Work out the finished part from the listing and answer in its coordinate system (mm). Face numbers are marked on the shaded views. A direction names the side the tool comes from. Coordinates: 2 decimals unless noted, no trailing zeros. Order: outer loops, then holes, each group sorted by start corner. A loop starts at its lowest first (then second) coordinate and runs counter-clockwise, first axis right, second up. Notation, with made-up numbers: M 75.5,44 L 105.5,44 A19 ccw 105.5,70 Z; hole C -24.75,65.25 d8. An arc over 180 degrees is marked long. Use a Markdown table: item, result.
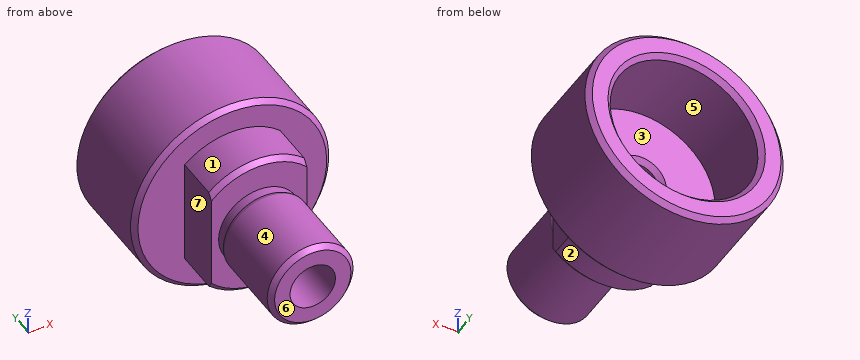
from build123d import *

# Parameters (mm, degrees)
CHAFL_N1_SIZE         = 1
REDONDEO1_R           = 1
CHAFL_N2_SIZE         = 1
CROQUIS3_W            = 14.730869345
CROQUIS3_H            = 22.360679774
CORTAR_EXTRUIR1_DEPTH = 30


with BuildPart() as part:
    # Croquis1 → Revolución1 (revolve)
    with BuildSketch(Plane.XY, mode=Mode.PRIVATE) as revoluci_n1_sk:
        Polygon((15.5, 52), (20.790206312, 52), (20.790206312, 30), (15, 30), (15, 20), (8.5, 20), (8.5, 17.951688966), (9, 17.951688966), (9, 0), (4.7625, 0), (4.7625, 30), (4.2625, 30), (4.2625, 34), (5.2625, 35), (15.5, 35), align=None)
    revolve(revoluci_n1_sk.sketch.rotate(Axis((0, 50.374990084, 0), (0, -1, 0)), 90), axis=Axis((0, 50.374990084, 0), (0, -1, 0)))

    # Chaflán1
    chafl_n1_edges = [part.edges().sort_by_distance(p)[0] for p in [
        (0, 0, -9),
    ]]
    chamfer(chafl_n1_edges, length=CHAFL_N1_SIZE)

    # Redondeo1
    # the kernel refuses this fillet: 1 mm, written as the material it takes off along each edge
    with BuildSketch(Plane(origin=(0, 17.951688966, 0), x_dir=(0, 0, 1), z_dir=(1, 0, 0))) as redondeo1_piece_1:
        with BuildLine():
            CenterArc((8, 0.866025404), REDONDEO1_R, 300, 60)
            Line((8.5, 0), (8.51, -0.017320508))
            ThreePointArc((8.51, -0.017320508), (8.75, -0.02), (9, -0.02))
            Line((9, -0.02), (9.02, 0))
            Line((9.02, 0), (9.02, 0.866025404))
            Line((9.02, 0.866025404), (9, 0.866025404))
        make_face()
    revolve(axis=Axis((0, 17.951688966, 0), (0, -1, 0)), mode=Mode.SUBTRACT)

    # Chaflán2
    chafl_n2_edges = [part.edges().sort_by_distance(p)[0] for p in [
        (0, 20, -15),
        (0, 30, -20.790206312),
        (0, 52, -20.790206312),
        (0, 52, -15.5),
    ]]
    chamfer(chafl_n2_edges, length=CHAFL_N2_SIZE)

    # Croquis3 → Cortar-Extruir1 (cut)
    with BuildSketch(Plane.XZ):
        Polygon((10, 11.180339887), (10, -11.180339887), (24.245950338, -11.180339887), (24.827853146, 11.180339887), align=None)
        with Locations((-17.365434673, 0)):
            Rectangle(CROQUIS3_W, CROQUIS3_H)
    extrude(amount=-CORTAR_EXTRUIR1_DEPTH, mode=Mode.SUBTRACT)


solid = part.part
(1) Which of the six approach directions +Z, -Z, +X, -X, +Y, -Y give full straight-line access (tool end or side, diameter ignored) to the marked faces 1, 2, 3 and 4?
Conclusion:
| item | result |
|---|---|
| face 1 | +Z, -Y |
| face 2 | -Z, -Y |
| face 3 | +Y |
| face 4 | -Y |
(2) Given P1, Ø6, axis at y = 10.5, z = -5, coming from the +X side; P2, Ø4, axis at y = 44, z = 13, coming from the -X side; P3, Ø11, axis at y = 24, z = 2, coming from the +X side, each flat-ended and moving along its own axis, determine where each tip first touches the part or whether it passes through.
Conclusion:
| item | result |
|---|---|
| P1 | x = 8.77 |
| P2 | x = -17.64 |
| P3 | x = 10 |
(3) Straight lines are drawn through the part: L1, parallel to X at y = 23, z = 0; L2, parallel to X at y = 14.25, z = 0; L3, parallel to Y at x = 9.5, z = 5.5. For each, find the intervals that lie inside material, in ascending order.
Conclusion:
| item | result |
|---|---|
| L1 | -10 to -4.76, 4.76 to 10 |
| L2 | -9 to -4.76, 4.76 to 9 |
| L3 | 20 to 35 |
(4) Determine the mould class of the marked faces 5, 6 and 7 for opening direction X: pulls with the +X half, pulls with the -X half, needs draft (parallel to the pull), parting line crosses it, or undercut.
Conclusion:
| item | result |
|---|---|
| face 5 | undercut |
| face 6 | needs draft |
| face 7 | pulls with the -X half |
(5) A cutting plane is placed at A-A (y = 36). Determine the outline of the cut face in (x, z).
Conclusion:
| item | result |
|---|---|
| outline | C 0,0 d41.58; hole C 0,0 d31 |
